Build history of the part. All positions in model axes, mm. Face numbers are marked on the shaded views. A direction names the side the tool comes from. Give positions to 0.01 mm unless a question says otherwise; leave off trailing zeros. Order: outer loops, then holes, each group sorted by start corner. A loop starts at its lowest first (then second) coordinate and runs counter-clockwise, first axis right, second up. Notation, with made-up numbers: (-17, -24.5) -> (5, -24.5) arc R18 ccw to (5, -12.5) -> close; hole circle Ø6 at (35.5, 18). An arc over 180 degrees is marked (long way). One line per question, with ' | ' between items. Start each with the question number.
(1) Pin check, flat tips, straight feed: pin 1 Ø1 at (x, z) = (2.5, 1) entering from -Y; pin 2 Ø1.5 at (x, z) = (-2.5, 1) entering from +Y; pin 3 Ø0.5 at (y, z) = (-2.5, -0.5) entering from +X. Stop position of each tip, or through.
(2) Drill centre lines: L1, parallel to Y at x = -2, z = 1.1; L2, parallel to Y at x = 1.75, z = 1.6; L3, parallel to Z at x = -6, y = 0.5. Where is each one in solid material? Low to high. Write a range as from..to.
(3) Cut at A-A (z = 0.5). Give the cut face in (x, y), then the cut area to 3 significant figures.
(4) Cut at B-B (x = 2.75). Give the cut face in (y, z).
(5) Which spindle directions (+Z, -Z, +X, -X, +Y, -Y) get a long thin tool onto all of the face, cutting with end or side? Do the marked faces 1, 2, 3 and 4. Say none if no direction does.
(6) Cut at C-C (y = 7). Give the cut face in (x, z), then the cut area to 3 significant figures.
(7) Cut at D-D (x = -2.1). Give the cut face in (y, z).
from build123d import *

# Parameters (mm, degrees)
SKETCH_1_W             = 13
SKETCH_1_H             = 23
EXTRUDE_1_DEPTH        = 1
SKETCH_2_W             = 1
SKETCH_2_H             = 20.6
CUT_EXTRUDE_1_DEPTH    = 0.1
CUT_EXTRUDE_3_REACH    = 15.248
PATTERN_LINEAR_8_COUNT = 4
PATTERN_LINEAR_8_PITCH = 1.4
MIRROR_3_COPY_1_REACH  = 15.248
MIRROR_3_COPY_2_REACH  = 15.248
MIRROR_3_COPY_3_REACH  = 15.248
CUT_EXTRUDE_4_REACH    = 15.248
PATTERN_LINEAR_9_COUNT = 8
PATTERN_LINEAR_9_PITCH = 1.4
MIRROR_4_COPY_1_REACH  = 15.248
MIRROR_4_COPY_2_REACH  = 15.248
MIRROR_4_COPY_3_REACH  = 15.248
MIRROR_4_COPY_4_REACH  = 15.248
MIRROR_4_COPY_5_REACH  = 15.248
MIRROR_4_COPY_6_REACH  = 15.248
MIRROR_4_COPY_7_REACH  = 15.248
SKETCH_12_W            = 10.9
SKETCH_12_H            = 11.68
EXTRUDE_2_DEPTH        = 1.9
CHAMFER_1_SIZE         = 1
CHAMFER_2_SIZE         = 1
SKETCH_13_W            = 6
SKETCH_13_H            = 8
EXTRUDE_3_DEPTH        = 1.27


with BuildPart() as part:
    # 草图1 → 凸台-拉伸1 (new body)
    with BuildSketch(Plane.XY):
        Rectangle(SKETCH_1_W, SKETCH_1_H)
    extrude(amount=-EXTRUDE_1_DEPTH)

    # 草图2 → 切除-拉伸1 (cut)
    with BuildSketch(Plane(origin=(6.5, 0, 0), x_dir=(0, 0, -1), z_dir=(1, 0, 0))):
        with Locations((0.5, -0.25)):
            Rectangle(SKETCH_2_W, SKETCH_2_H)
    cut_extrude_1 = extrude(amount=-CUT_EXTRUDE_1_DEPTH, mode=Mode.SUBTRACT)

    # 镜向1: 切除-拉伸1 across plane
    add(cut_extrude_1.mirror(Plane.ZY), mode=Mode.SUBTRACT)

    # 草图5 → 切除-拉伸3 (cut, up to next)
    with BuildSketch(Plane.XY, mode=Mode.PRIVATE) as cut_extrude_3_sk1:
        with BuildLine():
            Line((0.3, -11.5), (1.1, -11.5))
            ThreePointArc((1.1, -11.5), (0.7, -11.1), (0.3, -11.5))
        make_face()
    cut_extrude_3_tool1 = extrude(cut_extrude_3_sk1.sketch, amount=-CUT_EXTRUDE_3_REACH, mode=Mode.PRIVATE) & part.part
    cut_extrude_3 = cut_extrude_3_tool1.solids().sort_by_distance((0.7, -11.330235, 0))[0]
    add(cut_extrude_3, mode=Mode.SUBTRACT)

    # 阵列(线性)8: 切除-拉伸3 ×4
    with Locations(*[(i * PATTERN_LINEAR_8_PITCH, 0, 0) for i in range(1, PATTERN_LINEAR_8_COUNT)]):
        add(cut_extrude_3, mode=Mode.SUBTRACT)

    # 镜向3: 切除-拉伸3 across plane
    add(cut_extrude_3.mirror(Plane.ZY), mode=Mode.SUBTRACT)

    # 镜向3 copy 1 sketch → 镜向3 copy 1 (cut, up to next)
    with BuildSketch(Plane(origin=(-1.4, 0, 0), x_dir=(-1, 0, 0), z_dir=(0, 0, 1)), mode=Mode.PRIVATE) as mirror_3_copy_1_sk1:
        with BuildLine():
            Line((0.3, 11.5), (1.1, 11.5))
            ThreePointArc((1.1, 11.5), (0.7, 11.1), (0.3, 11.5))
        make_face()
    mirror_3_copy_1_tool1 = extrude(mirror_3_copy_1_sk1.sketch, amount=-MIRROR_3_COPY_1_REACH, mode=Mode.PRIVATE) & part.part
    add(mirror_3_copy_1_tool1.solids().sort_by_distance((-2.1, -11.330235, 0))[0], mode=Mode.SUBTRACT)

    # 镜向3 copy 2 sketch → 镜向3 copy 2 (cut, up to next)
    with BuildSketch(Plane(origin=(-2.8, 0, 0), x_dir=(-1, 0, 0), z_dir=(0, 0, 1)), mode=Mode.PRIVATE) as mirror_3_copy_2_sk1:
        with BuildLine():
            Line((0.3, 11.5), (1.1, 11.5))
            ThreePointArc((1.1, 11.5), (0.7, 11.1), (0.3, 11.5))
        make_face()
    mirror_3_copy_2_tool1 = extrude(mirror_3_copy_2_sk1.sketch, amount=-MIRROR_3_COPY_2_REACH, mode=Mode.PRIVATE) & part.part
    add(mirror_3_copy_2_tool1.solids().sort_by_distance((-3.5, -11.330235, 0))[0], mode=Mode.SUBTRACT)

    # 镜向3 copy 3 sketch → 镜向3 copy 3 (cut, up to next)
    with BuildSketch(Plane(origin=(-4.2, 0, 0), x_dir=(-1, 0, 0), z_dir=(0, 0, 1)), mode=Mode.PRIVATE) as mirror_3_copy_3_sk1:
        with BuildLine():
            Line((0.3, 11.5), (1.1, 11.5))
            ThreePointArc((1.1, 11.5), (0.7, 11.1), (0.3, 11.5))
        make_face()
    mirror_3_copy_3_tool1 = extrude(mirror_3_copy_3_sk1.sketch, amount=-MIRROR_3_COPY_3_REACH, mode=Mode.PRIVATE) & part.part
    add(mirror_3_copy_3_tool1.solids().sort_by_distance((-4.9, -11.330235, 0))[0], mode=Mode.SUBTRACT)

    # 草图11 → 切除-拉伸4 (cut, up to next)
    with BuildSketch(Plane.XY, mode=Mode.PRIVATE) as cut_extrude_4_sk1:
        with BuildLine():
            Line((-6.4, -8.55), (-6.4, -9.35))
            ThreePointArc((-6.4, -9.35), (-6, -8.95), (-6.4, -8.55))
        make_face()
    cut_extrude_4_tool1 = extrude(cut_extrude_4_sk1.sketch, amount=-CUT_EXTRUDE_4_REACH, mode=Mode.PRIVATE) & part.part
    cut_extrude_4 = cut_extrude_4_tool1.solids().sort_by_distance((-6.230235, -8.95, 0))[0]
    add(cut_extrude_4, mode=Mode.SUBTRACT)

    # 阵列(线性)9: 切除-拉伸4 ×8
    with Locations(*[(0, i * PATTERN_LINEAR_9_PITCH, 0) for i in range(1, PATTERN_LINEAR_9_COUNT)]):
        add(cut_extrude_4, mode=Mode.SUBTRACT)

    # 镜向4: 切除-拉伸4 across plane
    add(cut_extrude_4.mirror(Plane.ZY), mode=Mode.SUBTRACT)

    # 镜向4 copy 1 sketch → 镜向4 copy 1 (cut, up to next)
    with BuildSketch(Plane(origin=(0, 1.4, 0), x_dir=(-1, 0, 0), z_dir=(0, 0, 1)), mode=Mode.PRIVATE) as mirror_4_copy_1_sk1:
        with BuildLine():
            Line((-6.4, 8.55), (-6.4, 9.35))
            ThreePointArc((-6.4, 9.35), (-6, 8.95), (-6.4, 8.55))
        make_face()
    mirror_4_copy_1_tool1 = extrude(mirror_4_copy_1_sk1.sketch, amount=-MIRROR_4_COPY_1_REACH, mode=Mode.PRIVATE) & part.part
    add(mirror_4_copy_1_tool1.solids().sort_by_distance((6.230235, -7.55, 0))[0], mode=Mode.SUBTRACT)

    # 镜向4 copy 2 sketch → 镜向4 copy 2 (cut, up to next)
    with BuildSketch(Plane(origin=(0, 2.8, 0), x_dir=(-1, 0, 0), z_dir=(0, 0, 1)), mode=Mode.PRIVATE) as mirror_4_copy_2_sk1:
        with BuildLine():
            Line((-6.4, 8.55), (-6.4, 9.35))
            ThreePointArc((-6.4, 9.35), (-6, 8.95), (-6.4, 8.55))
        make_face()
    mirror_4_copy_2_tool1 = extrude(mirror_4_copy_2_sk1.sketch, amount=-MIRROR_4_COPY_2_REACH, mode=Mode.PRIVATE) & part.part
    add(mirror_4_copy_2_tool1.solids().sort_by_distance((6.230235, -6.15, 0))[0], mode=Mode.SUBTRACT)

    # 镜向4 copy 3 sketch → 镜向4 copy 3 (cut, up to next)
    with BuildSketch(Plane(origin=(0, 4.2, 0), x_dir=(-1, 0, 0), z_dir=(0, 0, 1)), mode=Mode.PRIVATE) as mirror_4_copy_3_sk1:
        with BuildLine():
            Line((-6.4, 8.55), (-6.4, 9.35))
            ThreePointArc((-6.4, 9.35), (-6, 8.95), (-6.4, 8.55))
        make_face()
    mirror_4_copy_3_tool1 = extrude(mirror_4_copy_3_sk1.sketch, amount=-MIRROR_4_COPY_3_REACH, mode=Mode.PRIVATE) & part.part
    add(mirror_4_copy_3_tool1.solids().sort_by_distance((6.230235, -4.75, 0))[0], mode=Mode.SUBTRACT)

    # 镜向4 copy 4 sketch → 镜向4 copy 4 (cut, up to next)
    with BuildSketch(Plane(origin=(0, 5.6, 0), x_dir=(-1, 0, 0), z_dir=(0, 0, 1)), mode=Mode.PRIVATE) as mirror_4_copy_4_sk1:
        with BuildLine():
            Line((-6.4, 8.55), (-6.4, 9.35))
            ThreePointArc((-6.4, 9.35), (-6, 8.95), (-6.4, 8.55))
        make_face()
    mirror_4_copy_4_tool1 = extrude(mirror_4_copy_4_sk1.sketch, amount=-MIRROR_4_COPY_4_REACH, mode=Mode.PRIVATE) & part.part
    add(mirror_4_copy_4_tool1.solids().sort_by_distance((6.230235, -3.35, 0))[0], mode=Mode.SUBTRACT)

    # 镜向4 copy 5 sketch → 镜向4 copy 5 (cut, up to next)
    with BuildSketch(Plane(origin=(0, 7, 0), x_dir=(-1, 0, 0), z_dir=(0, 0, 1)), mode=Mode.PRIVATE) as mirror_4_copy_5_sk1:
        with BuildLine():
            Line((-6.4, 8.55), (-6.4, 9.35))
            ThreePointArc((-6.4, 9.35), (-6, 8.95), (-6.4, 8.55))
        make_face()
    mirror_4_copy_5_tool1 = extrude(mirror_4_copy_5_sk1.sketch, amount=-MIRROR_4_COPY_5_REACH, mode=Mode.PRIVATE) & part.part
    add(mirror_4_copy_5_tool1.solids().sort_by_distance((6.230235, -1.95, 0))[0], mode=Mode.SUBTRACT)

    # 镜向4 copy 6 sketch → 镜向4 copy 6 (cut, up to next)
    with BuildSketch(Plane(origin=(0, 8.4, 0), x_dir=(-1, 0, 0), z_dir=(0, 0, 1)), mode=Mode.PRIVATE) as mirror_4_copy_6_sk1:
        with BuildLine():
            Line((-6.4, 8.55), (-6.4, 9.35))
            ThreePointArc((-6.4, 9.35), (-6, 8.95), (-6.4, 8.55))
        make_face()
    mirror_4_copy_6_tool1 = extrude(mirror_4_copy_6_sk1.sketch, amount=-MIRROR_4_COPY_6_REACH, mode=Mode.PRIVATE) & part.part
    add(mirror_4_copy_6_tool1.solids().sort_by_distance((6.230235, -0.55, 0))[0], mode=Mode.SUBTRACT)

    # 镜向4 copy 7 sketch → 镜向4 copy 7 (cut, up to next)
    with BuildSketch(Plane(origin=(0, 9.8, 0), x_dir=(-1, 0, 0), z_dir=(0, 0, 1)), mode=Mode.PRIVATE) as mirror_4_copy_7_sk1:
        with BuildLine():
            Line((-6.4, 8.55), (-6.4, 9.35))
            ThreePointArc((-6.4, 9.35), (-6, 8.95), (-6.4, 8.55))
        make_face()
    mirror_4_copy_7_tool1 = extrude(mirror_4_copy_7_sk1.sketch, amount=-MIRROR_4_COPY_7_REACH, mode=Mode.PRIVATE) & part.part
    add(mirror_4_copy_7_tool1.solids().sort_by_distance((6.230235, 0.85, 0))[0], mode=Mode.SUBTRACT)

    # 草图12 → 凸台-拉伸2 (add)
    with BuildSketch(Plane.XY):
        with Locations((0, -4.61)):
            Rectangle(SKETCH_12_W, SKETCH_12_H)
    extrude(amount=EXTRUDE_2_DEPTH)

    # 倒角1
    chamfer_1_edges = [part.edges().sort_by_distance(p)[0] for p in [
        (5.45, 1.23, 0.95),
    ]]
    chamfer(chamfer_1_edges, length=CHAMFER_1_SIZE)

    # 倒角2
    chamfer_2_edges = [part.edges().sort_by_distance(p)[0] for p in [
        (-5.45, -10.45, 0.95),
    ]]
    chamfer(chamfer_2_edges, length=CHAMFER_2_SIZE)

    # 草图13 → 凸台-拉伸3 (add)
    with BuildSketch(Plane.XY):
        with Locations((0, 6.8)):
            Rectangle(SKETCH_13_W, SKETCH_13_H)
    extrude(amount=EXTRUDE_3_DEPTH)


solid = part.part
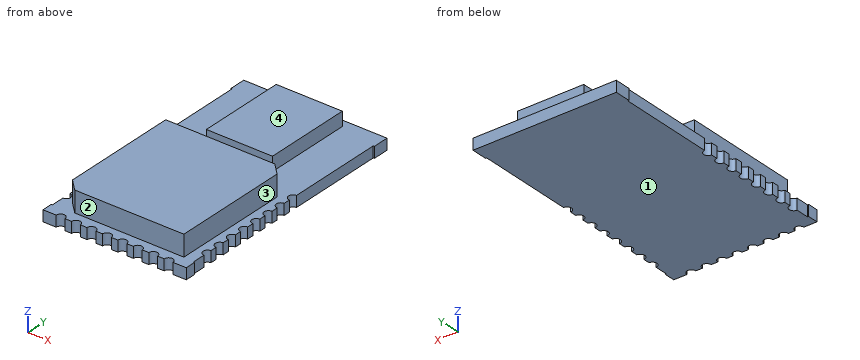
Result set:
1) pin 1: stops at y = -10.45 | pin 2: stops at y = 10.8 | pin 3: stops at x = 6.4
2) L1: y = -10.45..1.23, 2.8..10.8 | L2: y = -10.45..1.23 | L3: z = -1..0
3) outline: (-5.45, -9.45) -> (-4.45, -10.45) -> (5.45, -10.45) -> (5.45, 0.23) -> (4.45, 1.23) -> (-5.45, 1.23) -> close; (-3, 2.8) -> (3, 2.8) -> (3, 10.8) -> (-3, 10.8) -> close | area: 174 mm2
4) outline: (-11.5, -1) -> (11.5, -1) -> (11.5, 0) -> (10.8, 0) -> (10.8, 1.27) -> (2.8, 1.27) -> (2.8, 0) -> (1.23, 0) -> (1.23, 1.9) -> (-10.45, 1.9) -> (-10.45, 0) -> (-11.5, 0) -> close
5) face 1: -Z, +X, -X, +Y, -Y | face 2: +Z, +X, -X, -Y | face 3: +Z, +X, +Y, -Y | face 4: +Z, +X, -X, +Y
6) outline: (-6.4, -1) -> (6.4, -1) -> (6.4, 0) -> (3, 0) -> (3, 1.27) -> (-3, 1.27) -> (-3, 0) -> (-6.4, 0) -> close | area: 20.4 mm2
7) outline: (-11.1, -1) -> (11.5, -1) -> (11.5, 0) -> (10.8, 0) -> (10.8, 1.27) -> (2.8, 1.27) -> (2.8, 0) -> (1.23, 0) -> (1.23, 1.9) -> (-10.45, 1.9) -> (-10.45, 0) -> (-11.1, 0) -> close
